from build123d import *

# Parameters (mm, degrees)
BOSS_EXTRUDE1_DEPTH                           = 15
FILLET1_R                                     = 5
FILLET2_R                                     = 3
CSK_FOR_4_FLAT_HEAD_MACHINE_SCREW2_AT_2_COUNT = 2
CSK_FOR_4_FLAT_HEAD_MACHINE_SCREW2_AT_2_PITCH = 20


with BuildPart() as part:
    # Sketch1 → Boss-Extrude1 (new body, symmetric)
    with BuildSketch(Plane(origin=(0, 0, 0), x_dir=(0, 0, -1), z_dir=(1, 0, 0))):
        Polygon((-60, 0), (0, 0), (0, 55), (26, 55), (26, 63), (-8, 63), (-8, 8), (-53.5, 8), (-53.5, 23), (-60, 23), align=None)
    extrude(amount=BOSS_EXTRUDE1_DEPTH, both=True)

    # Fillet1
    fillet1_edges = [part.edges().sort_by_distance(p)[0] for p in [
        (0, 8, 8),
        (0, 63, 8),
        (0, 55, -26),
        (0, 0, 0),
        (0, 0, 60),
    ]]
    fillet(fillet1_edges, radius=FILLET1_R)

    # Fillet2
    fillet2_edges = [part.edges().sort_by_distance(p)[0] for p in [
        (0, 23, 60),
        (0, 23, 53.5),
        (0, 8, 53.5),
        (0, 55, 0),
    ]]
    fillet(fillet2_edges, radius=FILLET2_R)

    # Sketch6 → CSK for #4 Flat Head Machine Screw2 (revolve, cut)
    with BuildSketch(Plane(origin=(-10, 55, -13), x_dir=(0, 0, -1), z_dir=(1, 0, 0))):
        Polygon((0, 0), (0, 8), (1.63195, 8), (1.63195, 6.409835609), (2.857501397, 5), (2.857501397, 0), align=None)
    csk_for_4_flat_head_machine_screw2 = revolve(axis=Axis((-10, 48.65, -13), (0, 1, 0)), mode=Mode.SUBTRACT)

    # CSK for #4 Flat Head Machine Screw2 at 2: CSK for #4 Flat Head Machine Screw2 ×2
    with Locations(*[(i * CSK_FOR_4_FLAT_HEAD_MACHINE_SCREW2_AT_2_PITCH, 0, 0) for i in range(1, CSK_FOR_4_FLAT_HEAD_MACHINE_SCREW2_AT_2_COUNT)]):
        add(csk_for_4_flat_head_machine_screw2, mode=Mode.SUBTRACT)


solid = part.part
Here's how the part is built. I have some questions about the finished solid (model axes, mm). A direction names the side the tool comes from. Coordinates: 2 decimals unless noted, no trailing zeros. Write each loop counter-clockwise with the first axis right and the second up, starting at its lowest first coordinate (ties: lowest second). Pieces come first, ordered by that corner, then holes. Notation, with made-up numbers: (86.25, -23.5) - (115.25, -23.5) arc R22 ccw to (115.25, -1.5) - close; hole circle Ø4 at (34.5, 23). An arc over 180 degrees is marked (long way). Use one line per item in the form item = value.
1) Suppose I cut it at A-A, the plane y = 18. Write out the boundary of the cut face in (x, z), plus the area to 3 significant figures.
Solved:
outline = (-15, 0) - (15, 0) - (15, 8) - (-15, 8) - close; (-15, 53.5) - (15, 53.5) - (15, 60) - (-15, 60) - close
area = 435 mm2
2) Suppose I cut it at C-C, the plane z = -13. Write out the boundary of the cut face in (x, y).
Solved:
outline = (-15, 55) - (-12.86, 55) - (-12.86, 60) - (-11.63, 61.41) - (-11.63, 63) - (-15, 63) - close; (-8.37, 61.41) - (-7.14, 60) - (-7.14, 55) - (7.14, 55) - (7.14, 60) - (8.37, 61.41) - (8.37, 63) - (-8.37, 63) - close; (11.63, 61.41) - (12.86, 60) - (12.86, 55) - (15, 55) - (15, 63) - (11.63, 63) - close
3) On a 3-axis mill with a long thin cutter (end or side, diameter ignored), from which of +Z, -Z, +X, -X, +Y, -Y can I reach the whole of each face in a straight line? I mean faces 1 (the cylindrical face through (11.09, 57.46, -15.64)), 2 (the flat face through (0, 28, 0)), 3 (the cylindrical face through (0, 9, 10)). Say none if no direction works.
Solved:
face_1 = -Y
face_2 = -Z, +X, -X, -Y
face_3 = +X, -X, +Y
4) Thinking about a two-plate mould opening in Z: for faces 4 (the cylindrical face through (-7.465, 57.465, -14.319)), 5 (the flat face through (-15, 27, 7.6)), 6 (the cylindrical face through (0, 1, 58)), which applies, released by +Z, released by -Z, zero draft, split by the parting line, or undercut?
Solved:
face_4 = undercut
face_5 = zero draft
face_6 = released by +Z
5) I need wall thicknesses on line 1 (X direction, y = 62, z = -13); line 2 (X direction, y = 58.2, z = -13); line 3 (Z direction, x = 7.5, y = 28.5). Which ranges of each line are inside material? Lowest first, please.
Solved:
line_1 = -15 to -11.63, -8.37 to 8.37, 11.63 to 15
line_2 = -15 to -12.86, -7.14 to 7.14, 12.86 to 15
line_3 = 0 to 8
6) I'm going to push flat-ended pins straight in: P1, Ø2, axis at x = 6, y = 20.5, coming from the -Z side; P2, Ø9, axis at x = -10, z = -13, coming from the -Y side; P3, Ø6, axis at x = -2, z = 35, coming from the +Y side. Where does each tip first touch, or does it pass through?
Solved:
P1 = 0
P2 = 55
P3 = 8
7) Suppose I cut it at D-D, the plane x = -4.75. Write out the boundary of the cut face in (y, z).
Solved:
outline = (0, 5) arc R5 ccw to (5, 0) - (52, 0) arc R3 cw to (55, -3) - (55, -21) arc R5 ccw to (60, -26) - (63, -26) - (63, 3) arc R5 ccw to (58, 8) - (13, 8) arc R5 cw to (8, 13) - (8, 50.5) arc R3 cw to (11, 53.5) - (20, 53.5) arc R3 ccw to (23, 56.5) - (23, 57) arc R3 ccw to (20, 60) - (5, 60) arc R5 ccw to (0, 55) - close
8) Suppose I cut it at B-B, the plane x = -10. Write out the boundary of the cut face in (y, z).
Solved:
outline = (0, 5) arc R5 ccw to (5, 0) - (52, 0) arc R3 cw to (55, -3) - (55, -10.14) - (60, -10.14) - (61.41, -11.37) - (63, -11.37) - (63, 3) arc R5 ccw to (58, 8) - (13, 8) arc R5 cw to (8, 13) - (8, 50.5) arc R3 cw to (11, 53.5) - (20, 53.5) arc R3 ccw to (23, 56.5) - (23, 57) arc R3 ccw to (20, 60) - (5, 60) arc R5 ccw to (0, 55) - close; (55, -21) arc R5 ccw to (60, -26) - (63, -26) - (63, -14.63) - (61.41, -14.63) - (60, -15.86) - (55, -15.86) - close
